from build123d import *

# Parameters (mm, degrees)
F1_DEPTH    = 6
F2_DEPTH    = 0.8
F3_T1_DEPTH = 431.7925725323
F4_DEPTH    = 35


# Not quite as in the source:
# - a fillet or chamfer that OpenCascade refuses, or shapes differently, is made with other operations: its cross-section is extruded or revolved along the edge and cut away or added


with BuildPart() as f1:
    # F0 (on Top) → F1 (new body)
    with BuildSketch(Plane.XY):
        Polygon((150, 17.5), (-150, 17.5), (-150, -17.5), (150, -17.5), (150, -11.1123658717), (0, -11.1123658717), (0, -8.0123320222), (150, -8.0123320222), (150, 9.5545258373), (0, 9.5545258373), (0, 12.9128964618), (150, 12.9128964618), align=None)
    extrude(amount=F1_DEPTH)

    # F2 (add): faces of the model
    f2_faces = [f1.faces().sort_by_distance(p)[0] for p in [
        (-7.6230433236, -0.1272136786, 0),
        (-7.6230433236, -0.1272136786, 6),
    ]]
    extrude(f2_faces, amount=F2_DEPTH, dir=(0, 0, -1))

    # F3: fillet of radius 120.7106781187 on 1 edges, made by hand

    # F3_s2 → F3_t1 (cut)
    with BuildSketch(Plane.XY.offset(-213.2962862662)):
        with BuildLine():
            ThreePointArc((-65.0014854935, 17.5), (-110.9627394699, 8.4075593911), (-150, -17.5))
            Line((-150, -17.5), (-150, 17.5))
            Line((-150, 17.5), (-65.0014854935, 17.5))
        make_face()
    extrude(amount=F3_T1_DEPTH, mode=Mode.SUBTRACT)

    # F4 (cut): faces of the model
    f4_faces = [f1.faces().sort_by_distance(p)[0] for p in [
        (150, 15.2064482309, 2.6),
        (150, -14.3061829358, 2.6),
    ]]
    extrude(f4_faces, amount=-F4_DEPTH, mode=Mode.SUBTRACT)


solid = f1.part
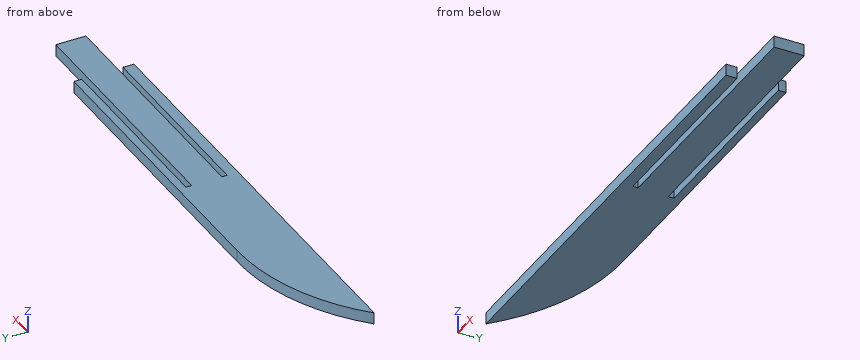
Read the model definition and answer for the solid it produces. Units are mm, in the model's axes. Coordinates: 2 decimals unless noted, no trailing zeros. Loops run counter-clockwise (first coordinate to the right, second up) from the corner with the lowest first, then second, coordinate; pieces in that order, holes last. Notation, with made-up numbers: (78, -40) -> (87, -40) arc R6 ccw to (87, -29) -> close; hole circle Ø8 at (-18.5, -38.75). An arc over 180 degrees is marked (long way). Answer in a Markdown table with one row per item.
Item 1: A cutting plane is placed at D-D on x = -125. Determine the outline of the cut face in (y, z).
Returned:
| item | result |
|---|---|
| outline | (-17.5, -0.8) -> (1.53, -0.8) -> (1.53, 6) -> (-17.5, 6) -> close |
Item 2: Straight lines are drawn through the part: line 1 along Y through (x, z) = (63, 2); line 2 along Y through (x, z) = (-74.5, 5.5); line 3 along X through (y, z) = (-12, 4.5). For each, find the intervals that lie inside material, in ascending order. Write a range as [from, to].
Returned:
| item | result |
|---|---|
| line 1 | y = [-17.5, -11.11], [-8.01, 9.55], [12.91, 17.5] |
| line 2 | y = [-17.5, 17.13] |
| line 3 | x = [-144.07, 115] |
Item 3: A cutting plane is placed at C-C on y = 4. Determine the outline of the cut face in (x, z), plus the area to 3 significant figures.
Returned:
| item | result |
|---|---|
| outline | (-120.47, -0.8) -> (150, -0.8) -> (150, 6) -> (-120.47, 6) -> close |
| area | 1,840 mm^2 |
Item 4: A cutting plane is placed at A-A on x = 99.5. Determine the outline of the cut face in (y, z).
Returned:
| item | result |
|---|---|
| outline | (-17.5, -0.8) -> (-11.11, -0.8) -> (-11.11, 6) -> (-17.5, 6) -> close; (-8.01, -0.8) -> (9.55, -0.8) -> (9.55, 6) -> (-8.01, 6) -> close; (12.91, -0.8) -> (17.5, -0.8) -> (17.5, 6) -> (12.91, 6) -> close |
Item 5: Each of these flat-tipped pins is pushed along its axis until it touches: P1, Ø1.4, axis at y = 15.5, z = 1, coming from the +X side; P2, Ø4, axis at x = 86.5, y = 12, coming from the +Z side. Where does it stop, or does it pass through?
Returned:
| item | result |
|---|---|
| P1 | stops at x = 115 |
| P2 | stops at z = 6 |
Item 6: A cutting plane is placed at B-B on z = 2. Determine the outline of the cut face in (x, y), plus the area to 3 significant figures.
Returned:
| item | result |
|---|---|
| outline | (-150, -17.5) -> (115, -17.5) -> (115, -11.11) -> (0, -11.11) -> (0, -8.01) -> (150, -8.01) -> (150, 9.55) -> (0, 9.55) -> (0, 12.91) -> (115, 12.91) -> (115, 17.5) -> (-65, 17.5) arc R120.71 ccw to start |
| area | 8,220 mm^2 |
